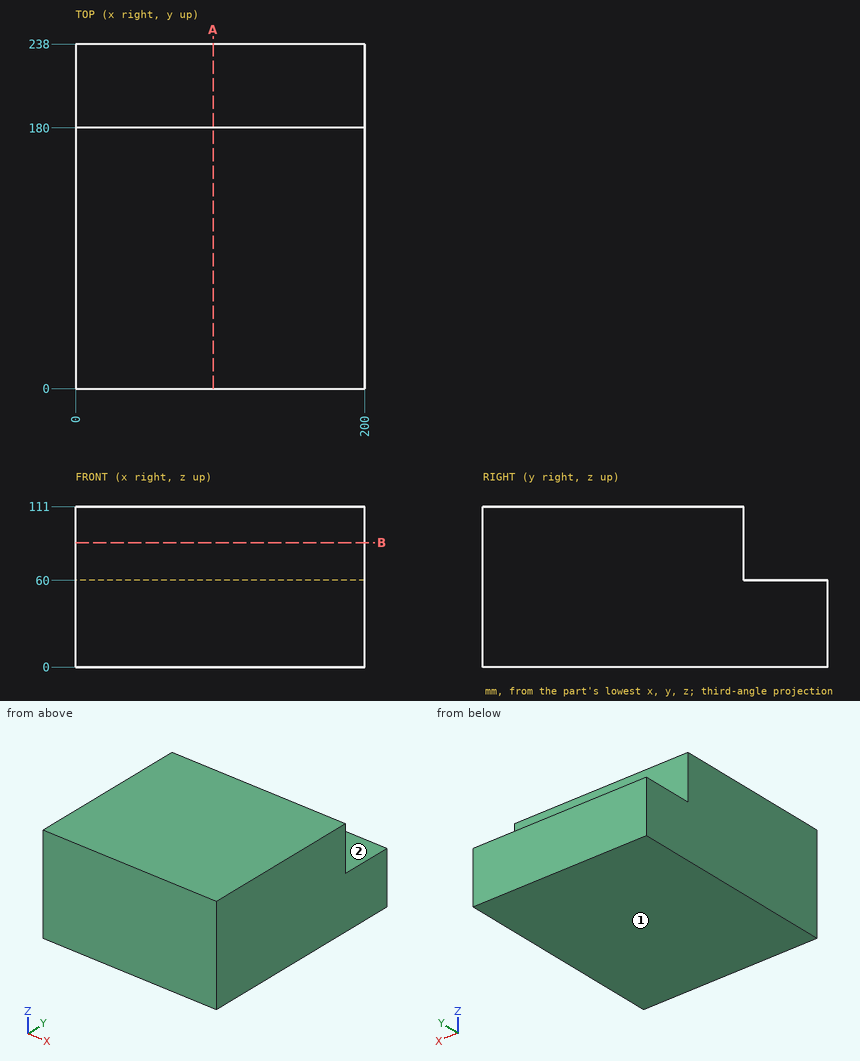
Part print with two shaded views. Sizes in mm from the minimum x, y, z corner. A direction names the side the tool comes from. Coordinates: 2 decimals unless noted, no trailing zeros. Write each loop counter-clockwise with the first axis right and the second up, starting at its lowest first coordinate (ties: lowest second). Pieces come first, ordered by that corner, then holes. Notation, with made-up numbers: (-31.75, -2) - (12.25, -2) arc R16 ccw to (12.25, 9) - close; hole circle Ø10 at (2, 18). An arc over 180 degrees is marked (long way). One line per item, written item: value. Start each with the question number.
1. Flat gauge pins, fed straight in: pin 1 (10 mm diameter, centred on x = 47, z = 68.5, fed in from +Y); pin 2 (4 mm diameter, centred on x = 147, y = 204.5, fed in from +Z); pin 3 (5 mm diameter, centred on y = 210, z = 62, fed in from +X). Where does each tip first touch, or does it go through?
2. Slice it at B-B (z = 86). Write the cut outline in (x, y).
3. Tool access for the marked faces 1 and 2: list every direction of +Z, -Z, +X, -X, +Y, -Y with a clear straight run to the whole face (end or side of a thin tool).
4. Slice it at A-A (x = 95). Write the cut outline in (y, z), plus the area to 3 significant figures.
5. Probe line 1 (Z direction, x = 104, y = 202); line 2 (Y direction, x = 77, z = 82). List the from-to ranges inside material, lowest first. Write a range as from..to.
Answers below:
1. pin 1: stops at y = 180
1. pin 2: stops at z = 60
1. pin 3: stops at x = 200
2. outline: (0, 0) - (200, 0) - (200, 180) - (0, 180) - close
3. face 1: -Z, +X, -X, +Y, -Y
3. face 2: +Z, +X, -X, +Y
4. outline: (0, 0) - (238, 0) - (238, 60) - (180, 60) - (180, 111) - (0, 111) - close
4. area: 23,500 mm^2
5. line 1: z = 0..60
5. line 2: y = 0..180
